Design review of the part built by this model. Coordinates are the model's own, in mm. A direction names the side the tool comes from. Coordinates: 2 decimals unless noted, no trailing zeros. Write each loop counter-clockwise with the first axis right and the second up, starting at its lowest first coordinate (ties: lowest second). Pieces come first, ordered by that corner, then holes.
Q1. Machinability: for faces 1 (the flat face through (-2, -4, 0)), 2 (the flat face through (0, 0, -3.48)), which of the approach directions +Z, -Z, +X, -X, +Y, -Y give a long, thin tool a straight path to every point of the face, cutting with its end or side? Answer none if there is none.
Q2. Take a section at C-C (z = -0.5). Give the boundary of the cut face in (x, y), and give its area (3 significant figures).
Q3. Insertion check: pin 1 (1 mm diameter, centred on y = 5, z = -1.5, fed in from +X); pin 2 (3 mm diameter, centred on y = -2.5, z = -0.5, fed in from +X). Each pin has a flat end and moves straight along its axis. Give the tip position at first contact, or say it passes through.
Q4. For probe 1 along Z at (x, y) = (2.25, 4); probe 2 along Z at (x, y) = (1, -5.5); probe 3 along X at (y, z) = (1, -1.25), list the stretches that pass through material, from the lowest coordinate up.
```python
from build123d import *

# Parameters (mm, degrees)
F0_R     = 4.0005
F1_DEPTH = 3.4798
F0_R_2   = 5.0165
F2_DEPTH = 1.397
F3_R     = 8.1534
F3_R_2   = 5.0165
F4_DEPTH = 1.27
F5_R     = 1.26999


# Not quite as in the source:
# - a fillet or chamfer is up to 0.001 mm smaller than in the source, because OpenCascade refuses the exact size


with BuildPart() as f1:
    # F0 (on Top) → F1 (new body)
    with BuildSketch(Plane.XY):
        Circle(F0_R)
    extrude(amount=-F1_DEPTH)

    # F0 (on Top) → F2 (join)
    with BuildSketch(Plane.XY):
        Circle(F0_R_2)
        Circle(F0_R, mode=Mode.SUBTRACT)
        Circle(F0_R)
    extrude(amount=F2_DEPTH)

    # F3 (on face) → F4 (join)
    with BuildSketch(Plane.XY.offset(1.397)):
        Circle(F3_R)
        Circle(F3_R_2, mode=Mode.SUBTRACT)
        Circle(F3_R_2)
    extrude(amount=F4_DEPTH)

    # F5 (radius 1.27 in the source; OpenCascade refuses exactly that, so slightly less here)
    f5_edges = [f1.edges().sort_by_distance(p)[0] for p in [
        (-8.1534, 0, 2.667),
    ]]
    fillet(f5_edges, radius=F5_R)


solid = f1.part
```
Response:
1. face 1: -Z
1. face 2: -Z, +X, -X, +Y, -Y
2. outline: circle Ø8 at (0, 0)
2. area: 50.3 mm2
3. pin 1: passes through
3. pin 2: stops at x = 4.9
4. probe 1: z = 0 to 2.67
4. probe 2: z = 1.4 to 2.67
4. probe 3: x = -3.87 to 3.87
